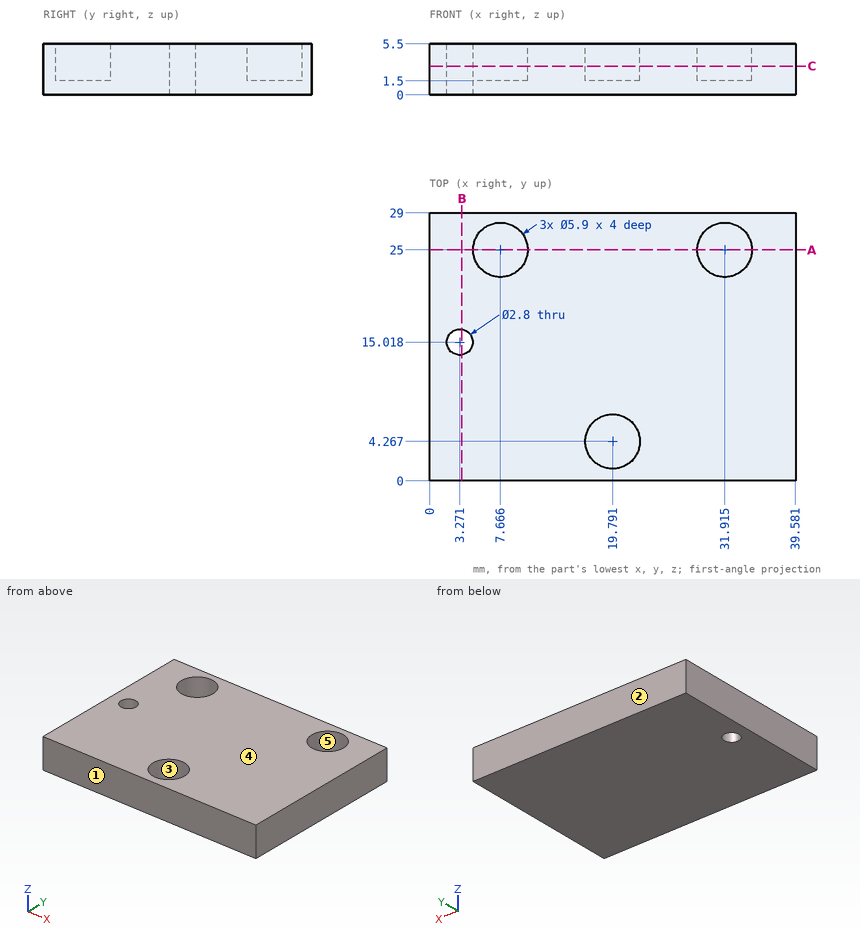
Drawing for the job (mm, zero at the part's lowest x, y, z). A direction names the side the tool comes from. Round coordinates to 2 decimals unless told otherwise and drop trailing zeros. Loops run counter-clockwise (first coordinate to the right, second up) from the corner with the lowest first, then second, coordinate; pieces in that order, holes last. Notation, with made-up numbers: (30, 22) -> (43, 22) arc R24 cw to (43, 48) -> close; hole circle Ø2 at (7.5, 39.25). An arc over 180 degrees is marked (long way). Answer in a Markdown table with one row per item.
Item 1: Drill centre lines: L1, parallel to X at y = 25, z = 4.7 (1 decimal); L2, parallel to X at y = 24, z = 2.5; L3, parallel to Y at x = 34.5, z = 4.8. Where is each one in solid material? Low to high. Write a range as [from, to].
Answers below:
| item | result |
|---|---|
| L1 | x = [0, 4.7], [10.6, 29], [34.9, 39.6] |
| L2 | x = [0, 4.89], [10.44, 29.14], [34.69, 39.58] |
| L3 | y = [0, 23.58], [26.42, 29] |
Item 2: Saw through at C-C (z = 3.1). State how many separate pieces and enclosed holes the cut face has, and give its area (3 significant figures).
Answers below:
| item | result |
|---|---|
| separate pieces | 1 |
| enclosed holes | 4 |
| area | 1,060 mm² |
Item 3: Mould opens along Y. For the marked faces 1, 2 and 3 say: +Y half, -Y half, draft (parallel to the pull), parting line (faces both ways), or undercut.
Answers below:
| item | result |
|---|---|
| face 1 | -Y half |
| face 2 | +Y half |
| face 3 | undercut |
Item 4: Pin check, flat tips, straight feed: pin 1 (3 mm diameter, centred on x = 20, y = 3.5, fed in from +Z); pin 2 (1.7 mm diameter, centred on x = 3.27, y = 15.02, fed in from +Z). Stop position of each tip, or through.
Answers below:
| item | result |
|---|---|
| pin 1 | stops at z = 1.5 |
| pin 2 | passes through |
Item 5: Saw through at A-A (y = 25). Write the cut outline in (x, z) (1 decimal).
Answers below:
| item | result |
|---|---|
| outline | (0, 0) -> (39.6, 0) -> (39.6, 5.5) -> (34.9, 5.5) -> (34.9, 1.5) -> (29, 1.5) -> (29, 5.5) -> (10.6, 5.5) -> (10.6, 1.5) -> (4.7, 1.5) -> (4.7, 5.5) -> (0, 5.5) -> close |
Item 6: Saw through at B-B (x = 3.5). Write the cut outline in (y, z), and give its area (3 significant figures).
Answers below:
| item | result |
|---|---|
| outline | (0, 0) -> (13.64, 0) -> (13.64, 5.5) -> (0, 5.5) -> close; (16.4, 0) -> (29, 0) -> (29, 5.5) -> (16.4, 5.5) -> close |
| area | 144 mm² |
Item 7: Which spindle directions (+Z, -Z, +X, -X, +Y, -Y) get a long thin tool onto all of the face, cutting with end or side? Do the marked faces 4 and 5. Say none if no direction does.
Answers below:
| item | result |
|---|---|
| face 4 | +Z, +X, -X, +Y, -Y |
| face 5 | +Z |
